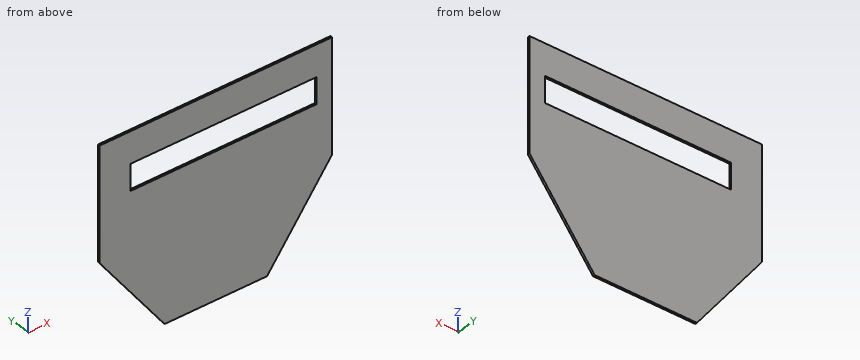
from build123d import *

# Parameters (mm, degrees)
EXTRUDE_1_DEPTH     = 4
CUT_EXTRUDE_1_REACH = 447.081
SKETCH_2_W          = 360
SKETCH_2_H          = 50


with BuildPart() as part:
    # 草图1 → 凸台-拉伸1 (new body)
    with BuildSketch(Plane(origin=(0, 0, 0), x_dir=(1, 0, 0), z_dir=(0, 1, 0))):
        Polygon((-225, 0), (225, 0), (225, 216), (99, 384), (-99, 384), (-225, 216), align=None)
    extrude(amount=EXTRUDE_1_DEPTH)

    # 草图2 → 切除-拉伸1 (cut, up to next)
    with BuildSketch(Plane(origin=(0, 4, 0), x_dir=(1, 0, 0), z_dir=(0, 1, 0)), mode=Mode.PRIVATE) as cut_extrude_1_sk1:
        with Locations((15, 85)):
            Rectangle(SKETCH_2_W, SKETCH_2_H)
    cut_extrude_1_tool1 = extrude(cut_extrude_1_sk1.sketch, amount=-CUT_EXTRUDE_1_REACH, mode=Mode.PRIVATE) & part.part
    add(cut_extrude_1_tool1.solids().sort_by_distance((15, 4, -85))[0], mode=Mode.SUBTRACT)


solid = part.part
Could you check a few things on this model? Use its own coordinates, in mm. Coordinates: 2 decimals unless noted, no trailing zeros. Order: outer loops, then holes, each group sorted by start corner. A loop starts at its lowest first (then second) coordinate and runs counter-clockwise, first axis right, second up.
Q1. Suppose I cut it at B-B on x = 162. Please give me the cut outline in (y, z).
Q2. Suppose I cut it at C-C on y = 1.7. Please give me the cut outline in (x, z), and give its area (3 significant figures).
Q3. Suppose I cut it at D-D on z = -337. Please give me the cut outline in (x, y).
Q4. Please list where these lines run through material, in increasing order: L1, parallel to X at y = 3.65, z = -67; L2, parallel to Z at x = -33, y = 1.3; L3, parallel to Z at x = 168.5, y = 1.55.
Q5. Suppose I cut it at A-A on z = -91.5. Please give me the cut outline in (x, y).
Q6. Will these pins go through, and if not, where does the flat tip stop? pin 1 (1.5 mm diameter, centred on x = 0, z = -335.5, fed in from -Y); pin 2 (1.5 mm diameter, centred on x = 101, y = 3, fed in from -Z).
Answer:
1. outline: (0, -300) - (4, -300) - (4, -110) - (0, -110) - close; (0, -60) - (4, -60) - (4, 0) - (0, 0) - close
2. outline: (-225, -216) - (-99, -384) - (99, -384) - (225, -216) - (225, 0) - (-225, 0) - close; hole (-165, -110) - (195, -110) - (195, -60) - (-165, -60) - close
2. area: 134,000 mm2
3. outline: (-134.25, 0) - (134.25, 0) - (134.25, 4) - (-134.25, 4) - close
4. L1: x = -225 to -165, 195 to 225
4. L2: z = -384 to -110, -60 to 0
4. L3: z = -291.33 to -110, -60 to 0
5. outline: (-225, 0) - (-165, 0) - (-165, 4) - (-225, 4) - close; (195, 0) - (225, 0) - (225, 4) - (195, 4) - close
6. pin 1: stops at y = 0
6. pin 2: stops at z = -382.33
